from build123d import *

# Parameters (mm, degrees)
F2_R          = 5.4088164631
F4_DEPTH      = 25.4
F4_DEPTH_BACK = 25.4


with BuildPart() as f3:
    # F0 (on Top) → F3 section 0
    with BuildSketch(Plane.XY, mode=Mode.PRIVATE) as f3_s0:
        Polygon((20.1203916222, 0), (0, 28.4514948726), (-18.8628677279, 0), align=None)
    loft([f3_s0.sketch, Vertex(0, 11.4749111235, 50.8)])

    # F2 (on offset) → F4 (join, two sides)
    with BuildSketch(Plane.XY.offset(50.8)) as f4_sk:
        with Locations((0, 11.4749111235)):
            Circle(F2_R)
    extrude(amount=F4_DEPTH)
    extrude(f4_sk.sketch, amount=-F4_DEPTH_BACK)

    # F5 (on face) → F6 (revolve)
    with BuildSketch(Plane.XY.offset(76.2)):
        with BuildLine():
            ThreePointArc((0, 2.5385186467), (6.3189837197, 5.1559274038), (8.9363924768, 11.4749111235))
            ThreePointArc((8.9363924768, 11.4749111235), (6.3189837197, 17.7938948432), (0, 20.4113036003))
            Line((0, 20.4113036003), (0, 16.8837275866))
            ThreePointArc((0, 16.8837275866), (3.8246107992, 15.2995219227), (5.4088164631, 11.4749111235))
            ThreePointArc((5.4088164631, 11.4749111235), (3.8246107992, 7.6503003243), (0, 6.0660946605))
            Line((0, 6.0660946605), (0, 2.5385186467))
        make_face()
    revolve(axis=Axis((0, 11.4749111235, 76.2), (0, -1, 0)))


solid = f3.part
Could you check a few things on this model? Use its own coordinates, in mm. Coordinates: 2 decimals unless noted, no trailing zeros. Write each loop counter-clockwise with the first axis right and the second up, starting at its lowest first coordinate (ties: lowest second). Pieces come first, ordered by that corner, then holes. Notation, with made-up numbers: (-12, 20) - (21, 20) arc R26 ccw to (21, 34) - close; hole circle Ø11 at (-33, 34.5). An arc over 180 degrees is marked (long way). Put each result on its own line as item: value. Start each with the question number.
Q1. I want a section at C-C on y = 23.25. Write out the boundary of the cut face in (x, z).
Q2. Please list where these lines run through material, in increasing order: L1, parallel to Z at x = 0, y = 8; L2, parallel to Y at x = 3, z = 76.5; L3, parallel to Y at x = 4, z = 22.
Q3. I want a section at B-B on x = 18. Write out the boundary of the cut face in (y, z).
Q4. I want a section at A-A on z = 42. Write out the boundary of the cut face in (x, y).
Q5. I'm going to push flat-ended pins straight in: P1, Ø10, axis at x = -5.5, z = 53, coming from the +Y side; P2, Ø6, axis at x = 0, y = 21, coming from the +Z side; P3, Ø3, axis at x = 0.5, z = 42, coming from the -Y side. Where does each tip first touch, or does it pass through?
Q6. Thinking about a two-plate mould opening in Z: for faces 1 (the cylindrical face through (-0.7, 16.84, 47.55)), 2 (the flat face through (1, 11, 0)), which applies, pulls with the +Z half, pulls with the -Z half, needs draft (parallel to the pull), parting line crosses it, or undercut?
Checks:
1. outline: (-3.45, 0) - (3.68, 0) - (0, 15.56) - close
2. L1: 0 to 76.2, 80.34 to 84.43
2. L2: 3.06 to 6.98, 15.97 to 19.89
2. L3: 4.97 to 15.44
3. outline: (0, 0) - (3, 0) - (1.21, 5.35) - close
4. outline: circle Ø10.82 at (0, 11.47)
5. P1: y = 16.86
5. P2: z = 82.31
5. P3: y = 6.07
6. face 1: undercut
6. face 2: pulls with the -Z half
